Here's how the part is built. I have some questions about the finished solid (model axes, mm). A direction names the side the tool comes from. Round coordinates to 2 decimals unless told otherwise and drop trailing zeros. Loops run counter-clockwise (first coordinate to the right, second up) from the corner with the lowest first, then second, coordinate; pieces in that order, holes last. Notation, with made-up numbers: (72.5, 33.5) - (131.5, 33.5) arc R16 cw to (131.5, 42.5) - close; hole circle Ø9 at (13.5, 72). An arc over 180 degrees is marked (long way). Return JSON: item names as keys, results as strings. Group by question number.
```python
from build123d import *

# Parameters (mm, degrees)
SKETCH1_R           = 1.5
BOSS_EXTRUDE1_DEPTH = 10
SKETCH2_R           = 2.5
BOSS_EXTRUDE2_DEPTH = 3
CUT_EXTRUDE2_DEPTH  = 1.27
CHAMFER1_SIZE       = 0.254
CUT_SWEEP4_PITCH    = 2
CUT_SWEEP4_HEIGHT   = 9.04
CUT_SWEEP4_RADIUS   = 1.259947043


with BuildPart() as part:
    # Sketch1 → Boss-Extrude1 (new body)
    with BuildSketch(Plane(origin=(0, 0, 0), x_dir=(1, 0, 0), z_dir=(0, 1, 0))):
        Circle(SKETCH1_R)
    extrude(amount=BOSS_EXTRUDE1_DEPTH)

    # Sketch2 → Boss-Extrude2 (add)
    with BuildSketch(Plane(origin=(0, 10, 0), x_dir=(-1, 0, 0), z_dir=(0, 1, 0))):
        Circle(SKETCH2_R)
    extrude(amount=BOSS_EXTRUDE2_DEPTH)

    # Sketch3 → Cut-Extrude2 (cut)
    with BuildSketch(Plane(origin=(0, 13, 0), x_dir=(1, 0, 0), z_dir=(0, 1, 0))):
        Polygon((2.000485358, 0), (1.000242679, 1.73247114), (-1.000242679, 1.73247114), (-2.000485358, 0), (-1.000242679, -1.73247114), (1.000242679, -1.73247114), align=None)
    extrude(amount=-CUT_EXTRUDE2_DEPTH, mode=Mode.SUBTRACT)

    # Chamfer1
    chamfer1_edges = [part.edges().sort_by_distance(p)[0] for p in [
        (-1.5, 0, 0),
    ]]
    chamfer(chamfer1_edges, length=CHAMFER1_SIZE)

    # Cut-Sweep4: sweep along a helix
    with BuildLine() as cut_sweep4_path:
        Helix(CUT_SWEEP4_PITCH, CUT_SWEEP4_HEIGHT, CUT_SWEEP4_RADIUS, center=(0, 0, 0), direction=(0, 1, 0))
    # Sketch6 → Cut-Sweep4 (sweep, cut)
    with BuildSketch(Plane(origin=(0, 0, 0), x_dir=(0, 0, -1), z_dir=(1, 0, 0))):
        Polygon((-1.263842547, 0), (-2.577025719, 0.570115155), (-2.41416834, -0.852192409), align=None)
    sweep(path=cut_sweep4_path.line, is_frenet=True, mode=Mode.SUBTRACT)


solid = part.part
```
Q1. For faces 4 (the flat face through (0, 12, -1.732)), 5 (the flat face through (0, 0, 0)), which set-ups out of +Z, -Z, +X, -X, +Y, -Y let a thin tool reach every point of the face, with its end or its side?
Q2. Please list where these lines run through material, in increasing order: line 1 (X direction, y = 11.25, z = 0.1); line 2 (Y direction, x = -1.95, z = 1.2); line 3 (Y direction, x = -0.1, z = -1.6).
Q3. Will these pins go through, and if not, where does the flat tip stop? pin 1 Ø3 at (x, y) = (0, 9.5) entering from +Z; pin 2 Ø1 at (x, y) = (0.5, 4) entering from +Z; pin 3 Ø3 at (x, y) = (-0.5, 6.5) entering from -Z.
Q4. If we mould it in two halves opening along X, with no side actions, what happens to faces 1 (the cylindrical face through (0.54, 11.48, -2.44)), 2 (the flat face through (0, 10, -2)), 3 (the flat face through (1.51, 12.37, -0.85))? For each: +X half, -X half, draft (parallel to the pull), parting line (faces both ways), or undercut.
Q5. Imagine slicing it at A-A, the plane z = -2. List the corners of the cut face in (x, y) for me.
Output values:
{
 "1": {"face 4": "+Y", "face 5": "+Z, -Z, +X, -X, -Y"},
 "2": {"line 1": "x = -2.5 to 2.5", "line 2": "y = 10 to 13", "line 3": "y = 10 to 11.73"},
 "3": {"pin 1": "stops at z = 2.5", "pin 2": "stops at z = 1.5", "pin 3": "stops at z = -1.5"},
 "4": {"face 1": "parting line", "face 2": "draft", "face 3": "undercut"},
 "5": {"outline": "(-1.5, 10) - (1.5, 10) - (1.5, 13) - (-1.5, 13) - close"}
}
